from build123d import *

# Parameters (mm, degrees)
SKETCH1_W           = 509
SKETCH1_H           = 500
BOSS_EXTRUDE1_DEPTH = 0.5
CUT_EXTRUDE4_DEPTH  = 10


with BuildPart() as part:
    # Sketch1 → Boss-Extrude1 (new body)
    with BuildSketch(Plane.XY):
        with Locations((254.5, 250)):
            Rectangle(SKETCH1_W, SKETCH1_H)
        with BuildLine():
            Line((481.865015679, 444.006934605), (481.865015679, 394.675474189))
            ThreePointArc((481.865015679, 394.675474189), (458.585000651, 371.395459161), (435.304985623, 394.675474189))
            Line((435.304985623, 394.675474189), (435.304985623, 444.006934605))
            ThreePointArc((435.304985623, 444.006934605), (458.585000651, 467.286949633), (481.865015679, 444.006934605))
        make_face(mode=Mode.SUBTRACT)
    extrude(amount=BOSS_EXTRUDE1_DEPTH)

    # Sketch8 → Cut-Extrude4 (cut)
    with BuildSketch(Plane.XY.offset(0.5)):
        with BuildLine():
            Line((77.785706476, 423.532533194), (98.958896901, 423.532533194))
            ThreePointArc((98.958896901, 423.532533194), (113.066279785, 409.425150311), (98.958896901, 395.317767427))
            Line((98.958896901, 395.317767427), (77.785706476, 395.317767427))
            ThreePointArc((77.785706476, 395.317767427), (63.678323592, 409.425150311), (77.785706476, 423.532533194))
        make_face()
    extrude(amount=-CUT_EXTRUDE4_DEPTH, mode=Mode.SUBTRACT)


solid = part.part
Geometry check sheet. Reference: the model listing, model coordinates, mm. A direction names the side the tool comes from. Give positions to 0.01 mm unless a question says otherwise; leave off trailing zeros. Write each loop counter-clockwise with the first axis right and the second up, starting at its lowest first coordinate (ties: lowest second). Pieces come first, ordered by that corner, then holes. Notation, with made-up numbers: (44, 70.25) - (58, 70.25) arc R19 cw to (58, 87.25) - close; hole circle Ø6 at (-38, 26.5). An arc over 180 degrees is marked (long way). Put each result on its own line as item: value.
1. Sectioned sample at A-A, the plane z = 0.25. Enter the section's corners in (x, y) (3 decimals).
Ans:
outline: (0, 0) - (509, 0) - (509, 500) - (0, 500) - close; hole (77.786, 395.318) - (98.959, 395.318) arc R14.107 ccw to (98.959, 423.533) - (77.786, 423.533) arc R14.107 ccw to start; hole (435.305, 394.675) arc R23.28 ccw to (481.865, 394.675) - (481.865, 444.007) arc R23.28 ccw to (435.305, 444.007) - close
2. Thickness scan on line 1 (X direction, y = 401, z = 0.45); line 2 (Y direction, x = 457.5, z = 0.1); line 3 (Y direction, x = 470, z = 0.4). Record the ranges inside material, lowest first.
Ans:
line 1: x = 0 to 66.47, 110.27 to 435.3, 481.87 to 509
line 2: y = 0 to 371.42, 467.26 to 500
line 3: y = 0 to 374.39, 464.3 to 500
3. Draft check along X on faces 3 (the cylindrical face through (458.07, 467.28, 0.25)), 4 (the cylindrical face through (63.68, 409.11, 0.25)), 5 (the flat face through (251, 254, 0.5)). Enter one of: +X half, -X half, draft (parallel to the pull), parting line (faces both ways), or undercut.
Ans:
face 3: undercut
face 4: undercut
face 5: draft
4. Set-up check for faces 1 (the cylindrical face through (113.063, 409.735, 0.254)), 2 (the flat face through (251, 254, 0)): record each of +Z, -Z, +X, -X, +Y, -Y from which the full face is reachable in a straight line by a thin tool's end or side.
Ans:
face 1: +Z, -Z
face 2: -Z, +X, -X, +Y, -Y
